Verification items for the finished model (mm, model axes). A direction names the side the tool comes from. Coordinates: 2 decimals unless noted, no trailing zeros. Order: outer loops, then holes, each group sorted by start corner. A loop starts at its lowest first (then second) coordinate and runs counter-clockwise, first axis right, second up. Notation, with made-up numbers: (66, -14) -> (107, -14) arc R14 cw to (107, 13) -> close; hole circle Ø10 at (-3, -32.75). An arc over 180 degrees is marked (long way). Write item = value, one per line. Start each with the question number.
1. Cross-section at A-A on y = -60. Record the cut outline in (x, z), plus the area to 3 significant figures.
2. Cross-section at C-C on z = 0. Record the cut outline in (x, y) (3 decimals), plus the area to 3 significant figures.
3. Cross-section at B-B on y = -80. Record the cut outline in (x, z), plus the area to 3 significant figures.
4. Go/stop test with flat-tipped pins: P1, Ø6.5, axis at x = -12.5, y = -20, coming from the -Z side; P2, Ø6.5, axis at x = -12.5, y = -40, coming from the +Z side; P3, Ø2, axis at x = 9, z = -17.5, coming from the -Y side; P4, Ø5.5, axis at x = -12.5, y = -80, coming from the +Z side. Record where each tip stops, or that it passes through.
5. Set-up check for faces 1 (the flat face through (20, -52, -22)), 2 (the cylindrical face through (3.47, -142.11, -23.6)), 3 (the flat face through (-5, -44, -25)): record each of +Z, -Z, +X, -X, +Y, -Y from which the full face is reachable in a straight line by a thin tool's end or side.
6. Release check for a two-part mould opening along Y. For faces 4 (the flat face through (0, -79, -20)), 5 (the cylindrical face through (3, -61, -25)) record: +Y half, -Y half, draft (parallel to the pull), parting line (faces both ways), or undercut.
7. Cross-section at D-D on z = -25. Give the number of separate pieces and of enclosed holes in the cut face, plus the area to 3 significant figures.
8. Thickness scan on line 1 along Z through (x, y) = (-15, -3.5); line 2 along Z through (x, y) = (-13, -125.5); line 3 along Y through (x, z) = (-12.5, -17). Record the ranges inside material, lowest first. Write a range as from..to.
from build123d import *

# Parameters (mm, degrees)
F0_W      = 40
F0_H      = 50
F0_R      = 2.074
F0_R_2    = 4.515
F1_DEPTH  = 10
F2_W      = 40
F2_H      = 10
F3_DEPTH  = 140
F4_SIZE   = 1
F5_SIZE   = 2
F6_W      = 10
F6_H      = 37
F7_DEPTH  = 10
F8_R      = 4.99999
F9_R      = 2.074
F10_DEPTH = 10
F11_R     = 2.074
F12_DEPTH = 10.001
F13_R     = 2.074
F14_DEPTH = 16
F15_SIZE  = 1
F16_SIZE  = 1
F17_W     = 5
F17_H     = 30
F18_DEPTH = 10.001
F19_R     = 2.49999
F20_R     = 2.074
F21_DEPTH = 40.001
F22_SIZE  = 2


# Not quite as in the source:
# - a fillet or chamfer is up to 0.001 mm smaller than in the source, because OpenCascade refuses the exact size


with BuildPart() as f1:
    # F0 (on Front) → F1 (new body)
    with BuildSketch(Plane.XZ):
        with Locations((0, -5)):
            Rectangle(F0_W, F0_H)
        with Locations((-15, -15)):
            Circle(F0_R, mode=Mode.SUBTRACT)
        with Locations((15, -15)):
            Circle(F0_R, mode=Mode.SUBTRACT)
        with Locations((-15, 15)):
            Circle(F0_R, mode=Mode.SUBTRACT)
        Circle(F0_R_2, mode=Mode.SUBTRACT)
        with Locations((15, 15)):
            Circle(F0_R, mode=Mode.SUBTRACT)
    extrude(amount=F1_DEPTH)

    # F2 (on face) → F3 (join)
    with BuildSketch(Plane.XZ.offset(10)):
        with Locations((0, -25)):
            Rectangle(F2_W, F2_H)
    extrude(amount=F3_DEPTH)

    # F4
    f4_edges = [f1.edges().sort_by_distance(p)[0] for p in [
        (-17.074, -10, 15),
        (12.926, -10, 15),
        (12.926, -10, -15),
        (-17.074, -10, -15),
    ]]
    chamfer(f4_edges, length=F4_SIZE)

    # F5
    f5_edges = [f1.edges().sort_by_distance(p)[0] for p in [
        (-4.515, -10, 0),
    ]]
    chamfer(f5_edges, length=F5_SIZE)

    # F6 (on face) → F7 (cut, through all)
    with BuildSketch(Plane.XY.offset(-20)):
        with Locations((0, -43.5)):
            Rectangle(F6_W, F6_H)
    extrude(amount=-F7_DEPTH, mode=Mode.SUBTRACT)

    # F8 (radius 5 in the source; OpenCascade refuses exactly that, so slightly less here)
    f8_edges = [f1.edges().sort_by_distance(p)[0] for p in [
        (5, -62, -25),
        (-5, -62, -25),
        (5, -25, -25),
        (-5, -25, -25),
    ]]
    fillet(f8_edges, radius=F8_R)

    # F9 (on face) → F10 (cut, through all)
    with BuildSketch(Plane.XY.offset(-20)):
        with Locations((-12.5, -140)):
            Circle(F9_R)
        with Locations((-12.5, -120)):
            Circle(F9_R)
        with Locations((-12.5, -100)):
            Circle(F9_R)
        with Locations((-12.5, -80)):
            Circle(F9_R)
        with Locations((-12.5, -60)):
            Circle(F9_R)
        with Locations((12.5, -60)):
            Circle(F9_R)
        with Locations((12.5, -80)):
            Circle(F9_R)
        with Locations((12.5, -100)):
            Circle(F9_R)
        with Locations((12.5, -140)):
            Circle(F9_R)
        with Locations((12.5, -120)):
            Circle(F9_R)
        with Locations((-12.5, -40)):
            Circle(F9_R)
        with Locations((-12.5, -20)):
            Circle(F9_R)
        with Locations((12.5, -40)):
            Circle(F9_R)
        with Locations((12.5, -20)):
            Circle(F9_R)
    extrude(amount=-F10_DEPTH, mode=Mode.SUBTRACT)

    # F11 (on face) → F12 (cut, through all)
    with BuildSketch(Plane.XY.offset(-20)):
        with Locations((0, -13.5)):
            Circle(F11_R)
        with Locations((0, -21.5)):
            Circle(F11_R)
    extrude(amount=-F12_DEPTH, mode=Mode.SUBTRACT)

    # F13 (on face) → F14 (cut)
    with BuildSketch(Plane.XZ.offset(150)):
        with Locations((-5, -25)):
            Circle(F13_R)
        with Locations((5, -25)):
            Circle(F13_R)
    extrude(amount=-F14_DEPTH, mode=Mode.SUBTRACT)

    # F15
    f15_edges = [f1.edges().sort_by_distance(p)[0] for p in [
        (-2.074, -21.5, -30),
        (-2.074, -13.5, -30),
    ]]
    chamfer(f15_edges, length=F15_SIZE)

    # F16
    f16_edges = [f1.edges().sort_by_distance(p)[0] for p in [
        (-14.574, -140, -20),
        (10.426, -140, -20),
        (10.426, -120, -20),
        (-14.574, -120, -20),
        (10.426, -100, -20),
        (-14.574, -100, -20),
        (10.426, -80, -20),
        (-14.574, -80, -20),
        (10.426, -60, -20),
        (-14.574, -60, -20),
        (-14.574, -40, -20),
        (10.426, -40, -20),
        (-10.426, -20, -25),
        (-14.574, -20, -20),
        (-14.574, -20, -30),
        (14.574, -20, -25),
        (10.426, -20, -20),
        (10.426, -20, -30),
    ]]
    chamfer(f16_edges, length=F16_SIZE)

    # F17 (on face) → F18 (cut, through all)
    with BuildSketch(Plane.XY.offset(-20)):
        with Locations((0, -129)):
            Rectangle(F17_W, F17_H)
    extrude(amount=-F18_DEPTH, mode=Mode.SUBTRACT)

    # F19 (radius 2.5 in the source; OpenCascade refuses exactly that, so slightly less here)
    f19_edges = [f1.edges().sort_by_distance(p)[0] for p in [
        (-2.5, -144, -25),
        (2.5, -144, -25),
        (-2.5, -114, -25),
        (2.5, -114, -25),
    ]]
    fillet(f19_edges, radius=F19_R)

    # F20 (on face) → F21 (cut, through all)
    with BuildSketch(Plane(origin=(-20, 0, 0), x_dir=(0, -1, 0), z_dir=(-1, 0, 0))):
        with Locations((125.5, -25)):
            Circle(F20_R)
    extrude(amount=-F21_DEPTH, mode=Mode.SUBTRACT)

    # F22
    f22_edges = [f1.edges().sort_by_distance(p)[0] for p in [
        (-20, -123.426, -25),
        (20, -123.426, -25),
    ]]
    chamfer(f22_edges, length=F22_SIZE)


solid = f1.part
Worked out:
q1.outline = (-20, -30) -> (-14.57, -30) -> (-14.57, -21) -> (-15.57, -20) -> (-20, -20) -> close; (-10.43, -30) -> (-4, -30) -> (-4, -20) -> (-9.43, -20) -> (-10.43, -21) -> close; (4, -30) -> (10.43, -30) -> (10.43, -21) -> (9.43, -20) -> (4, -20) -> close; (14.57, -30) -> (20, -30) -> (20, -20) -> (15.57, -20) -> (14.57, -21) -> close
q1.area = 235 mm²
q2.outline = (-20, -10) -> (-6.515, -10) -> (-4.515, -8) -> (-4.515, 0) -> (-20, 0) -> close; (4.515, -8) -> (6.515, -10) -> (20, -10) -> (20, 0) -> (4.515, 0) -> close
q2.area = 306 mm²
q3.outline = (-20, -30) -> (-14.57, -30) -> (-14.57, -21) -> (-15.57, -20) -> (-20, -20) -> close; (-10.43, -30) -> (10.43, -30) -> (10.43, -21) -> (9.43, -20) -> (-9.43, -20) -> (-10.43, -21) -> close; (14.57, -30) -> (20, -30) -> (20, -20) -> (15.57, -20) -> (14.57, -21) -> close
q3.area = 315 mm²
q4.P1 = -30
q4.P2 = -20
q4.P3 = -10
q4.P4 = -20.32
q5.face_1 = +Z, -Z, +X, +Y, -Y
q5.face_2 = -Y
q5.face_3 = +Z, -Z
q6.face_4 = draft
q6.face_5 = undercut
q7.separate_pieces = 2
q7.enclosed_holes = 17
q7.area = 5,000 mm²
q8.line_1 = -30..-17.07, -12.93..12.93, 17.07..20
q8.line_2 = -30..-27.07, -22.93..-20
q8.line_3 = -10..0
